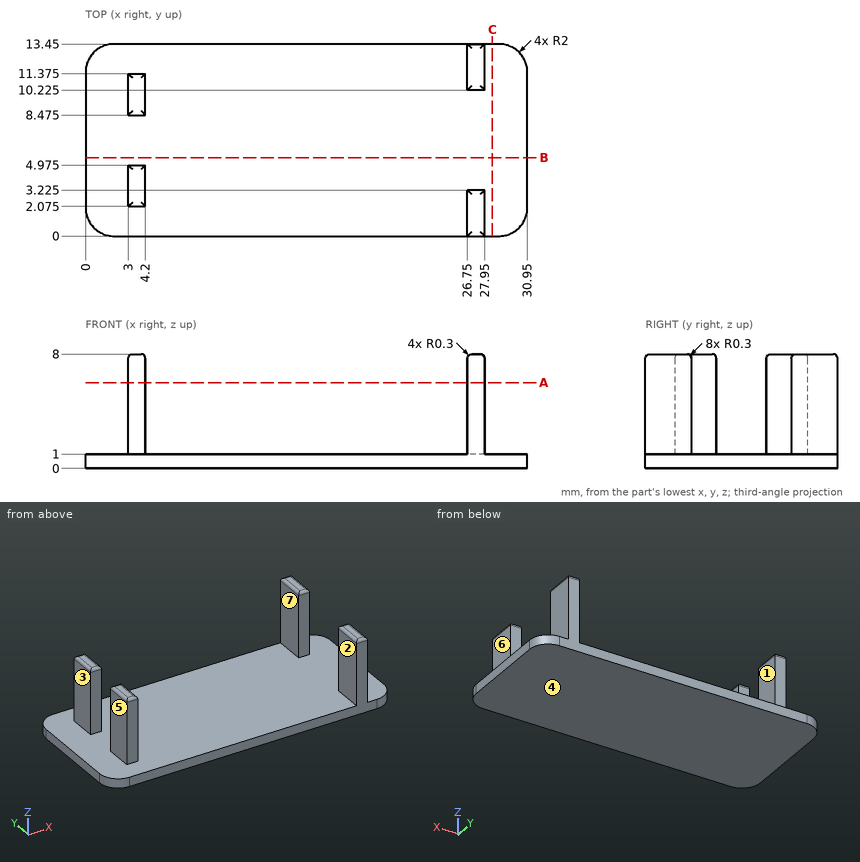
The figure shows three views and two pictorial views of one solid part (mm, origin at its lowest corner). Answer the questions. A direction names the side the tool comes from. Round coordinates to 2 decimals unless told otherwise and drop trailing zeros. Loops run counter-clockwise (first coordinate to the right, second up) from the corner with the lowest first, then second, coordinate; pieces in that order, holes last. Notation, with made-up numbers: M 16.5,51 L 63.5,51 A21 cw 63.5,64 Z; hole C 66.25,76.5 d7. An arc over 180 degrees is marked long. Return JSON: item names as keys, results as strings.
Q1. Find the intervals of material crossed by line 1 along X through (y, z) = (2.5, 2); line 2 along Z through (x, y) = (19.5, 7.75); line 3 along X through (y, z) = (4.5, 6.5), in increasing order. Write a range as from..to.
Results list:
{"line 1": "x = 3..4.2, 26.75..27.95", "line 2": "z = 0..1", "line 3": "x = 3..4.2"}
Q2. Find section A-A, the plane z = 6. Determine the outline of the cut face in (x, y) (3 decimals), plus the area to 3 significant figures.
Results list:
{"outline": "M 3,2.075 L 4.2,2.075 L 4.2,4.975 L 3,4.975 Z; M 3,8.475 L 4.2,8.475 L 4.2,11.375 L 3,11.375 Z; M 26.75,0 L 27.95,0 L 27.95,3.225 L 26.75,3.225 Z; M 26.75,10.225 L 27.95,10.225 L 27.95,13.45 L 26.75,13.45 Z", "area": "14.7 mm2"}
Q3. Which of the six approach directions +Z, -Z, +X, -X, +Y, -Y give full straight-line access (tool end or side, diameter ignored) to the marked faces 5, 6 and 7?
Results list:
{"face 5": "+Z, -X, +Y, -Y", "face 6": "+Z, +X, +Y, -Y", "face 7": "+Z, +Y, -Y"}
Q4. Find section C-C, the plane x = 28.5. Determine the outline of the cut face in (y, z), plus the area to 4 significant figures.
Results list:
{"outline": "M 0,0 L 13.45,0 L 13.45,1 L 0,1 Z", "area": "13.45 mm2"}
Q5. Find section B-B, the plane y = 5.5. Determine the outline of the cut face in (x, z), plus the area to 4 significant figures.
Results list:
{"outline": "M 0,0 L 30.95,0 L 30.95,1 L 0,1 Z", "area": "30.95 mm2"}
Q6. The mould has two halves that part along X. Classify the marked faces 1, 2, 3 and 4: released by +X, released by -X, zero draft, split by the parting line, or undercut.
Results list:
{"face 1": "undercut", "face 2": "undercut", "face 3": "released by -X", "face 4": "zero draft"}
Q7. Each of these flat-tipped pins is pushed along its axis until it touches: pin 1 Ø4 at (x, y) = (17, 11) entering from -Z; pin 2 Ø3 at (y, z) = (4, 5.5) entering from +X; pin 3 Ø3 at (y, z) = (11, 3) entering from -X; pin 4 Ø1.3 at (x, z) = (3.5, 5.5) entering from +Y (3 decimals). Where does it stop, or does it pass through?
Results list:
{"pin 1": "stops at z = 0", "pin 2": "stops at x = 27.95", "pin 3": "stops at x = 3", "pin 4": "stops at y = 11.375"}
